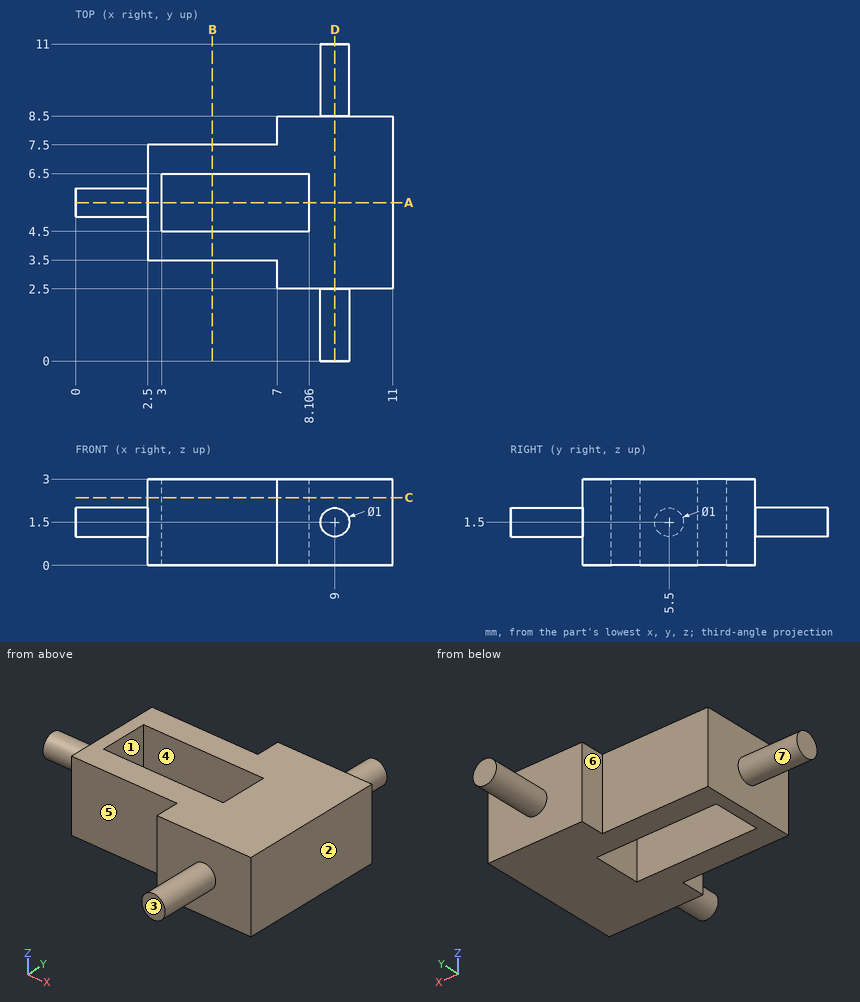
Here's the drawing with two shaded views (mm, measured from the low corner). I have some questions. A direction names the side the tool comes from. Give positions to 0.01 mm unless a question says otherwise; leave off trailing zeros. Write each loop counter-clockwise with the first axis right and the second up, starting at its lowest first coordinate (ties: lowest second). Pieces come first, ordered by that corner, then holes. Notation, with made-up numbers: (49.25, 43.5) - (75.25, 43.5) arc R27 cw to (75.25, 70.5) - close; hole circle Ø8 at (-27.5, 64.5). An arc over 180 degrees is marked (long way). Write item = value, one per line. Start each with the question number.
1. Imagine slicing it at D-D (x = 9). Please give me the cut outline in (y, z).
2. Please list where these lines run through material, in increasing order: line 1 (X direction, y = 5.5, z = 1.3); line 2 (Y direction, x = 6.5, z = 0.45); line 3 (Y direction, x = 8, z = 0.95).
3. For pin 1 (0.5 mm diameter, centred on y = 8, z = 2, fed in from -X); pin 2 (1.5 mm diameter, centred on y = 4.5, z = 2, fed in from -X); pin 3 (1.5 mm diameter, centred on x = 2.5, z = 2, fed in from +Y), each with a flat end and sliding along its axis, tell me the tip position at first contact or that it passes through.
4. Imagine slicing it at C-C (z = 2.35). Please give me the cut outline in (x, y), and give its area (3 significant figures).
5. On a 3-axis mill with a long thin cutter (end or side, diameter ignored), from which of +Z, -Z, +X, -X, +Y, -Y can I reach the whole of each face in a straight line? I mean the marked faces 5, 6 and 7. Say none if no direction works.
6. Thinking about a two-plate mould opening in X: for the marked faces 1, 2, 3 and 4, which applies, released by +X, released by -X, zero draft, split by the parting line, or undercut?
7. Imagine slicing it at A-A (y = 5.5). Please give me the cut outline in (x, z), and give its area (3 significant figures).
8. Imagine slicing it at B-B (x = 4.75). Please give me the cut outline in (y, z).
Worked answers:
q1.outline = (0, 1) - (2.5, 1) - (2.5, 0) - (8.5, 0) - (8.5, 1) - (11, 1) - (11, 2) - (8.5, 2) - (8.5, 3) - (2.5, 3) - (2.5, 2) - (0, 2) - close
q2.line_1 = 0 to 3, 8.11 to 11
q2.line_2 = 3.5 to 4.5, 6.5 to 7.5
q2.line_3 = 2.5 to 4.5, 6.5 to 8.5
q3.pin_1 = 7
q3.pin_2 = 0
q3.pin_3 = 7.5
q4.outline = (2.5, 3.5) - (7, 3.5) - (7, 2.5) - (11, 2.5) - (11, 8.5) - (7, 8.5) - (7, 7.5) - (2.5, 7.5) - close; hole (3, 4.5) - (8.11, 4.5) - (8.11, 6.5) - (3, 6.5) - close
q4.area = 31.8 mm2
q5.face_5 = +Z, -Z, -X, -Y
q5.face_6 = +Z, -Z, -X, +Y
q5.face_7 = -X
q6.face_1 = undercut
q6.face_2 = released by +X
q6.face_3 = zero draft
q6.face_4 = undercut
q7.outline = (0, 1) - (2.5, 1) - (2.5, 0) - (3, 0) - (3, 3) - (2.5, 3) - (2.5, 2) - (0, 2) - close; (8.11, 0) - (11, 0) - (11, 3) - (8.11, 3) - close
q7.area = 12.7 mm2
q8.outline = (3.5, 0) - (4.5, 0) - (4.5, 3) - (3.5, 3) - close; (6.5, 0) - (7.5, 0) - (7.5, 3) - (6.5, 3) - close
